For this review, take the finished solid that the model builds, in its own axes (mm). Face numbers are marked on the shaded views. A direction names the side the tool comes from. Give positions to 0.01 mm unless a question says otherwise; leave off trailing zeros. Order: outer loops, then holes, each group sorted by start corner. A loop starts at its lowest first (then second) coordinate and runs counter-clockwise, first axis right, second up. Notation, with made-up numbers: (-6, -2) -> (15, -2) arc R12 cw to (15, 3) -> close; hole circle Ø8 at (20.25, -2.75). An arc over 180 degrees is marked (long way). Return JSON: item names as keys, results as strings. Group by question number.
1) The part is to be moulded in two halves that separate along X. For the marked faces 3, 4 and 5, say which applies: released by +X, released by -X, zero draft, split by the parting line, or undercut.
2) Add section A-A (z = 18.25). Give the boundary of the cut face in (x, y) (3 decimals).
3) To check wall thickness, follow line 1 along Y through (x, z) = (-39.5, 4.25); line 2 along X through (y, z) = (-22.5, 4) (3 decimals). State the ranges of each line that lie inside material, in increasing order.
4) For the marked faces 1 and 2, list the 3-axis set-ups (+Z, -Z, +X, -X, +Y, -Y) from which the entire face can be reached by the end or side of a thin tool; tool diameter is ignored.
5) Add section B-B (y = -1). Give the boundary of the cut face in (x, z) (3 decimals), then the cut area to 4 significant figures.
6) Add section D-D (y = -24). Give the boundary of the cut face in (x, z) (3 decimals), then the cut area to 4 significant figures.
7) Add section C-C (x = 8.5). Give the boundary of the cut face in (y, z), then the cut area to 3 significant figures.
8) Insertion check: P1, Ø1.6, axis at x = 50.5, z = 10, coming from the +Y side; P2, Ø3, axis at x = 11, y = 23, coming from the +Z side; P3, Ø0.5, axis at x = 50, y = -30, coming from the +Z side. Each pin has a flat end and moves straight along its axis. Give the tip position at first contact, or say it passes through.
from build123d import *

# Parameters (mm, degrees)
F0_W      = 103.75
F0_H      = 64.5
F1_DEPTH  = 22
F2_T      = -2
F3_W      = 15
F3_H      = 7
F4_DEPTH  = 381
F5_R      = 2
F6_W      = 4.5
F6_H      = 9.5
F7_DEPTH  = 12.7
F8_R      = 2
F9_DEPTH  = 22
F10_R     = 2
F11_DEPTH = 20
F12_R     = 2
F13_DEPTH = 20
F14_R     = 2
F15_DEPTH = 22
F16_R     = 0.8
F17_DEPTH = 5.6
F18_R     = 0.8
F19_DEPTH = 5.6
F20_R     = 0.8
F21_DEPTH = 5.6
F22_R     = 0.8
F23_DEPTH = 5.6


with BuildPart() as f1:
    # F0 (on Top) → F1 (new body)
    with BuildSketch(Plane.XY):
        Rectangle(F0_W, F0_H)
    extrude(amount=F1_DEPTH)

    # F2
    f2_openings = [f1.faces().sort_by_distance(p)[0] for p in [
        (0, 0, 22),
    ]]
    offset(amount=F2_T, openings=f2_openings)

    # F3 (on Right) → F4 (cut)
    with BuildSketch(Plane.YZ):
        with Locations((0, 9)):
            Rectangle(F3_W, F3_H)
    extrude(amount=F4_DEPTH, mode=Mode.SUBTRACT)

    # F5
    f5_edges = [f1.edges().sort_by_distance(p)[0] for p in [
        (-51.875, 32.25, 11),
        (-51.875, -32.25, 11),
        (51.875, -32.25, 11),
        (51.875, 32.25, 11),
    ]]
    fillet(f5_edges, radius=F5_R)

    # F6 (on Top) → F7 (cut, symmetric)
    with BuildSketch(Plane.XY):
        with Locations((13.673813, 12.159993)):
            Rectangle(F6_W, F6_H)
    extrude(amount=F7_DEPTH, both=True, mode=Mode.SUBTRACT)

    # F8 (on Top) → F9 (join)
    with BuildSketch(Plane.XY):
        with Locations((-49.875, 30.25)):
            Circle(F8_R)
    extrude(amount=F9_DEPTH)

    # F10 (on face) → F11 (join)
    with BuildSketch(Plane.XY.offset(2)):
        with Locations((-49.875, -30.25)):
            Circle(F10_R)
    extrude(amount=F11_DEPTH)

    # F12 (on face) → F13 (join)
    with BuildSketch(Plane.XY.offset(2)):
        with Locations((49.875, -30.25)):
            Circle(F12_R)
    extrude(amount=F13_DEPTH)

    # F14 (on Top) → F15 (join)
    with BuildSketch(Plane.XY):
        with Locations((49.875, 30.25)):
            Circle(F14_R)
    extrude(amount=F15_DEPTH)

    # F16 (on face) → F17 (cut)
    with BuildSketch(Plane.XY.offset(22)):
        with Locations((-49.875, 30.25)):
            Circle(F16_R)
    extrude(amount=-F17_DEPTH, mode=Mode.SUBTRACT)

    # F18 (on face) → F19 (cut)
    with BuildSketch(Plane.XY.offset(22)):
        with Locations((-49.875, -30.25)):
            Circle(F18_R)
    extrude(amount=-F19_DEPTH, mode=Mode.SUBTRACT)

    # F20 (on face) → F21 (cut)
    with BuildSketch(Plane.XY.offset(22)):
        with Locations((49.875, -30.25)):
            Circle(F20_R)
    extrude(amount=-F21_DEPTH, mode=Mode.SUBTRACT)

    # F22 (on face) → F23 (cut)
    with BuildSketch(Plane.XY.offset(22)):
        with Locations((49.875, 30.25)):
            Circle(F22_R)
    extrude(amount=-F23_DEPTH, mode=Mode.SUBTRACT)


solid = f1.part
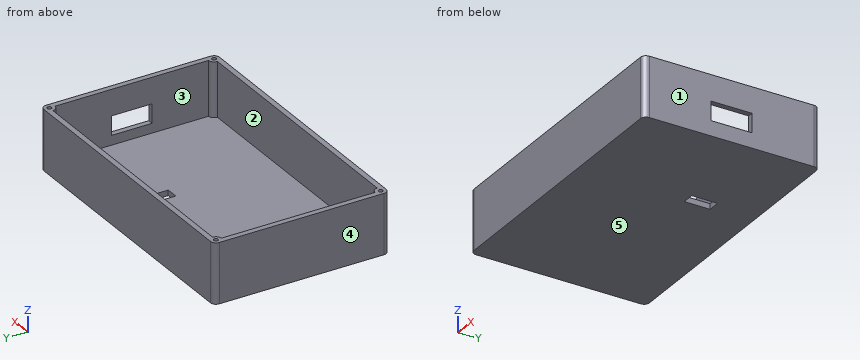
Evaluation:
{
 "1": {"face 3": "undercut", "face 4": "released by -X", "face 5": "zero draft"},
 "2": {"outline": "(-51.875, -30.25) arc R2 ccw to (-49.875, -32.25) -> (49.875, -32.25) arc R2 ccw to (51.875, -30.25) -> (51.875, 30.25) arc R2 ccw to (49.875, 32.25) -> (-49.875, 32.25) arc R2 ccw to (-51.875, 30.25) -> close; hole circle Ø1.6 at (-49.875, -30.25); hole circle Ø1.6 at (-49.875, 30.25); hole (-49.875, -28.25) arc R2 cw to (-47.875, -30.25) -> (47.875, -30.25) arc R2 cw to (49.875, -28.25) -> (49.875, 28.25) arc R2 cw to (47.875, 30.25) -> (-47.875, 30.25) arc R2 cw to (-49.875, 28.25) -> close; hole circle Ø1.6 at (49.875, -30.25); hole circle Ø1.6 at (49.875, 30.25)"},
 "3": {"line 1": "-32.25 to -30.25, 30.25 to 32.25", "line 2": "-51.875 to -49.875, 49.875 to 51.875"},
 "4": {"face 1": "+Z, -Z, +X, +Y, -Y", "face 2": "+Z"},
 "5": {"outline": "(-51.875, 0) -> (51.875, 0) -> (51.875, 5.5) -> (49.875, 5.5) -> (49.875, 2) -> (-49.875, 2) -> (-49.875, 22) -> (-51.875, 22) -> close; (49.875, 12.5) -> (51.875, 12.5) -> (51.875, 22) -> (49.875, 22) -> close", "area": "273.5 mm^2"},
 "6": {"outline": "(-51.875, 0) -> (51.875, 0) -> (51.875, 22) -> (49.875, 22) -> (49.875, 2) -> (-49.875, 2) -> (-49.875, 22) -> (-51.875, 22) -> close", "area": "287.5 mm^2"},
 "7": {"outline": "(-32.25, 0) -> (32.25, 0) -> (32.25, 22) -> (30.25, 22) -> (30.25, 2) -> (-30.25, 2) -> (-30.25, 22) -> (-32.25, 22) -> close", "area": "209 mm^2"},
 "8": {"P1": "y = 32.25", "P2": "z = 2", "P3": "z = 16.4"}
}
